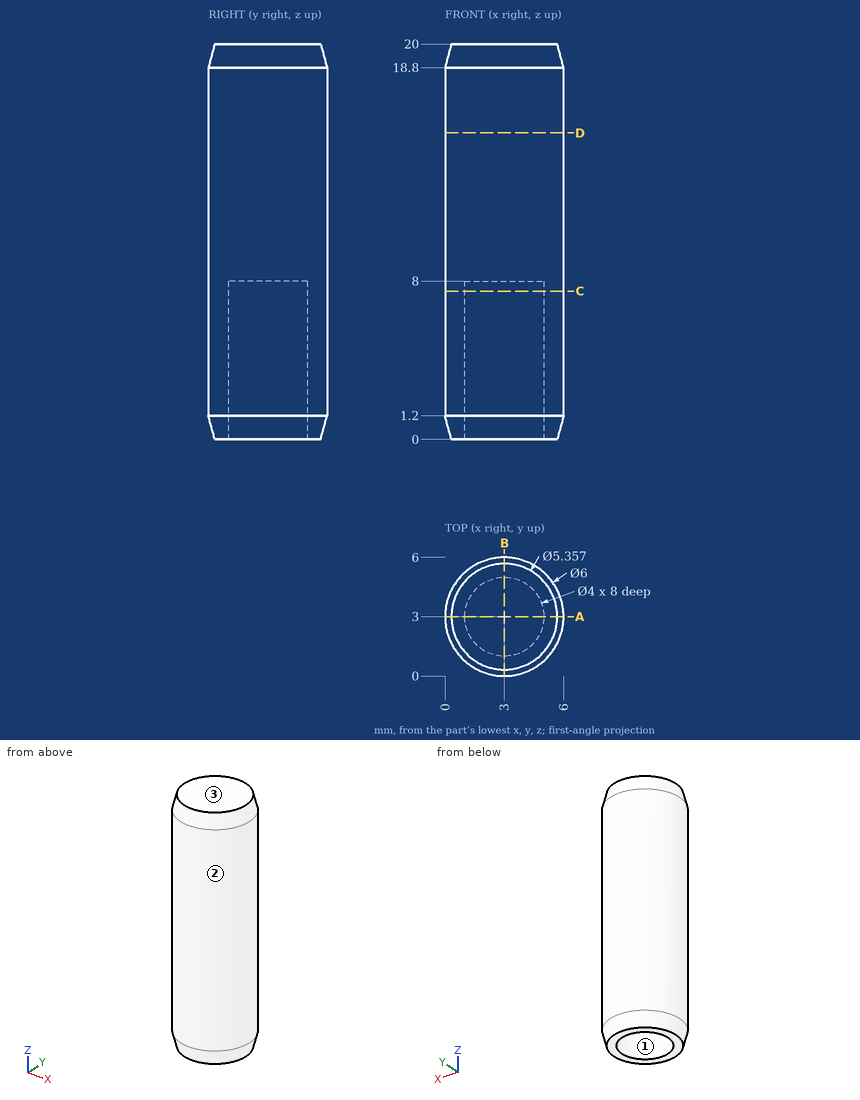
Input: dimensioned drawing with shaded views. Units: mm. Origin: part minimum x, y, z. Coordinates: 2 decimals unless noted, no trailing zeros. Loops run counter-clockwise (first coordinate to the right, second up) from the corner with the lowest first, then second, coordinate; pieces in that order, holes last. Notation, with made-up numbers: M 88.25,30.25 L 125.25,30.25 A12 ccw 125.25,48.25 Z; hole C -34,70.5 d3. An arc over 180 degrees is marked long. Put each result on its own line as item: value.
(1) Cut plane C-C on z = 7.5. Return the cut outline in (x, y), then the cut area to 3 significant figures.
Answer sheet:
outline: C 3,3 d6; hole C 3,3 d4
area: 15.7 mm^2
(2) Draft query along X for the marked faces 1, 2 and 3. Return one class per face: pulls with the +X half, pulls with the -X half, needs draft (parallel to the pull), parting line crosses it, or undercut.
Answer sheet:
face 1: undercut
face 2: parting line crosses it
face 3: needs draft
(3) Material intervals for probe 1 along Y at (x, z) = (3, 5.25); probe 2 along Z at (x, y) = (2.05, 2.75); probe 3 along Y at (x, z) = (3.6, 3.75), sorted ascending.
Answer sheet:
probe 1: y = 0 to 1, 5 to 6
probe 2: z = 8 to 20
probe 3: y = 0.06 to 1.09, 4.91 to 5.94
(4) Cut plane D-D on z = 15.5. Return the cut outline in (x, y), then the cut area to 3 significant figures.
Answer sheet:
outline: C 3,3 d6
area: 28.3 mm^2
(5) Cut plane A-A on y = 3. Return the cut outline in (x, z), then the cut area to 3 significant figures.
Answer sheet:
outline: M 0,1.2 L 0.32,0 L 1,0 L 1,8 L 5,8 L 5,0 L 5.68,0 L 6,1.2 L 6,18.8 L 5.68,20 L 0.32,20 L 0,18.8 Z
area: 87.2 mm^2
(6) First-contact query: pin 1 (1.5 mm diameter, centred on x = 1.5, z = 7.5, fed in from +Y); pin 2 (2 mm diameter, centred on x = 5, z = 8, fed in from -Y); pin 3 (3.5 mm diameter, centred on x = 3, y = 3, fed in from -Z). Flat tips, straight axial feed; report the tip coordinate or a pass-through.
Answer sheet:
pin 1: stops at y = 5.9
pin 2: stops at y = 0.17
pin 3: stops at z = 8
